```python
from build123d import *

# Parameters (mm, degrees)
SKETCH1_W           = 30.1625
SKETCH1_H           = 25.4
BOSS_EXTRUDE1_DEPTH = 15.875
SKETCH2_R           = 4.7625
BOSS_EXTRUDE2_DEPTH = 11.90625
SKETCH3_W           = 4.7625
SKETCH3_H           = 4.7625
CUT_EXTRUDE1_DEPTH  = 16.875


with BuildPart() as part:
    # Sketch1 → Boss-Extrude1 (new body)
    with BuildSketch(Plane(origin=(0, 0, 0), x_dir=(0, 0, -1), z_dir=(1, 0, 0))):
        Rectangle(SKETCH1_W, SKETCH1_H)
    extrude(amount=BOSS_EXTRUDE1_DEPTH)

    # Sketch2 → Boss-Extrude2 (add)
    with BuildSketch(Plane.XY.offset(15.08125)):
        with Locations((7.9375, 3.175)):
            Circle(SKETCH2_R)
    extrude(amount=BOSS_EXTRUDE2_DEPTH)

    # Sketch3 → Cut-Extrude1 (cut, through all)
    with BuildSketch(Plane(origin=(15.875, 0, 0), x_dir=(0, 0, -1), z_dir=(1, 0, 0))):
        with Locations((-12.7, -10.31875)):
            Rectangle(SKETCH3_W, SKETCH3_H)
    extrude(amount=-CUT_EXTRUDE1_DEPTH, mode=Mode.SUBTRACT)


solid = part.part
```
Verification items for the finished model (mm, model axes). A direction names the side the tool comes from. Round coordinates to 2 decimals unless told otherwise and drop trailing zeros. Order: outer loops, then holes, each group sorted by start corner. A loop starts at its lowest first (then second) coordinate and runs counter-clockwise, first axis right, second up.
1) Tool access check on faces 1 (the cylindrical face through (12.337, 1.351, 20.951)), 2 (the flat face through (0, 0, 0)), 3 (the flat face through (8, -7.938, 13)). Record the directions out of +Z, -Z, +X, -X, +Y, -Y that give a thin tool (end or side, any length) a straight path to the whole face; none if there is none.
Geometry says:
face 1: +Z
face 2: +Z, -Z, -X, +Y, -Y
face 3: +Z, +X, -X, -Y
2) Depth check by flat-ended pin: pin 1 (2.5 mm diameter, centred on x = 5, z = 12.5, fed in from -Y); pin 2 (1.5 mm diameter, centred on x = 3, y = 7.5, fed in from +Z); pin 3 (4 mm diameter, centred on x = 10, z = 18.5, fed in from -Y). Enter the tip coordinate at first touch or a pass-through.
Geometry says:
pin 1: stops at y = -7.94
pin 2: stops at z = 15.08
pin 3: stops at y = -1.59
3) Cross-section at A-A, the plane x = 5. Record the cut outline in (y, z).
Geometry says:
outline: (-12.7, -15.08) - (12.7, -15.08) - (12.7, 15.08) - (6.92, 15.08) - (6.92, 26.99) - (-0.57, 26.99) - (-0.57, 15.08) - (-7.94, 15.08) - (-7.94, 10.32) - (-12.7, 10.32) - close
4) Cross-section at D-D, the plane y = -4.25. Record the cut outline in (x, z) (3 decimals), plus the area to 3 significant figures.
Geometry says:
outline: (0, -15.081) - (15.875, -15.081) - (15.875, 15.081) - (0, 15.081) - close
area: 479 mm2
5) Cross-section at B-B, the plane y = -9. Record the cut outline in (x, z) (3 decimals).
Geometry says:
outline: (0, -15.081) - (15.875, -15.081) - (15.875, 10.319) - (0, 10.319) - close
6) Material ranges on line 1 (Z direction, x = 15.25, y = 4); line 2 (Y direction, x = 7, z = 15); line 3 (Y direction, x = 8.75, z = 23), recorded low to high.
Geometry says:
line 1: z = -15.08 to 15.08
line 2: y = -7.94 to 12.7
line 3: y = -1.52 to 7.87
7) Cross-section at C-C, the plane z = 24.5. Record the cut outline in (x, y) (1 decimal).
Geometry says:
outline: circle Ø9.5 at (7.9, 3.2)
